Build history of the part. All positions in model axes, mm. Round coordinates to 2 decimals unless told otherwise and drop trailing zeros. Write each loop counter-clockwise with the first axis right and the second up, starting at its lowest first coordinate (ties: lowest second). Pieces come first, ordered by that corner, then holes. Notation, with made-up numbers: (29, -4) -> (53, -4) arc R23 cw to (53, 33) -> close; hole circle Ø3 at (23, 57). An arc over 180 degrees is marked (long way). Answer as CSV lines item,"result".
from build123d import *

# Parameters (mm, degrees)
BOSS_EXTRUDE1_START     = 92.868812
BOSS_EXTRUDE1_DEPTH     = 3.175
FILLET1_R               = 9.525
F_1_4_CLEARANCE_HOLE1_D = 6.7564


with BuildPart() as part:
    # Sketch2 → Boss-Extrude1 (new body)
    with BuildSketch(Plane(origin=(0, 0, 0), x_dir=(0, 0, -1), z_dir=(1, 0, 0)).offset(BOSS_EXTRUDE1_START)):
        with BuildLine():
            Line((-1159.986800073, 353.698023512), (-1134.923032257, 357.817191252))
            Line((-1134.923032257, 357.817191252), (-1092.891252047, 364.725009516))
            Line((-1092.891252047, 364.725009516), (-1111.090669966, 321.220387339))
            Line((-1111.090669966, 321.220387339), (-1120.893160292, 297.788119344))
            ThreePointArc((-1120.893160292, 297.788119344), (-1128.752566193, 291.984337623), (-1137.588017099, 296.1543437))
            Line((-1137.588017099, 296.1543437), (-1166.34986848, 338.989401064))
            ThreePointArc((-1166.34986848, 338.989401064), (-1167.184141053, 348.080982608), (-1159.986800073, 353.698023512))
        make_face()
    extrude(amount=BOSS_EXTRUDE1_DEPTH)

    # Fillet1
    fillet1_edges = [part.edges().sort_by_distance(p)[0] for p in [
        (94.456312, 364.725009516, 1092.891252047),
    ]]
    fillet(fillet1_edges, radius=FILLET1_R)

    # 1/4 Clearance Hole1 (through all)
    with Locations(Plane(origin=(96.043812484, 0, 0), x_dir=(0, 0, -1), z_dir=(1, 0, 0))):
        with Locations((-1133.378344355, 348.418278321), (-1158.442112171, 344.299110581), (-1129.68026079, 301.464053216), (-1119.877770464, 324.896321212)):
            Hole(F_1_4_CLEARANCE_HOLE1_D / 2)


solid = part.part
1. Probe line 1 along Z through (x, y) = (95.4, 346.5); line 2 along Z through (x, y) = (94.7, 348); line 3 along Y through (x, z) = (95.75, 1135.5). List the from-to ranges inside material, lowest first.
Results found:
line 1,"z = 1100.52 to 1130.6, 1136.16 to 1155.88, 1161 to 1167.71"
line 2,"z = 1099.89 to 1130.03, 1136.73 to 1167.22"
line 3,"y = 293.92 to 345.79, 351.05 to 357.72"
2. Cut at D-D, the plane z = 1131.5. Write the cut outline in (x, y).
Results found:
outline,"(92.87, 292.11) -> (96.04, 292.11) -> (96.04, 298.62) -> (92.87, 298.62) -> close; (92.87, 304.31) -> (96.04, 304.31) -> (96.04, 345.61) -> (92.87, 345.61) -> close; (92.87, 351.23) -> (96.04, 351.23) -> (96.04, 358.38) -> (92.87, 358.38) -> close"
3. Cut at B-B, the plane y = 350.5. Write the cut outline in (x, z), then the cut area to 3 significant figures.
Results found:
outline,"(92.87, 1099.01) -> (96.04, 1099.01) -> (96.04, 1130.72) -> (92.87, 1130.72) -> close; (92.87, 1136.04) -> (96.04, 1136.04) -> (96.04, 1165.67) -> (92.87, 1165.67) -> close"
area,"195 mm2"
4. Drop flat-ended pins along their axis: pin 1 Ø6 at (y, z) = (348.42, 1133.38) entering from +X; pin 2 Ø1 at (x, y) = (93, 317) entering from +Z. Give the stop position or say it passes through.
Results found:
pin 1,"passes through"
pin 2,"stops at z = 1151.92"
5. Cut at A-A, the plane z = 1156. Write the cut outline in (x, y), then the cut area to 3 significant figures.
Results found:
outline,"(92.87, 323.58) -> (96.04, 323.58) -> (96.04, 341.96) -> (92.87, 341.96) -> close; (92.87, 346.63) -> (96.04, 346.63) -> (96.04, 354.35) -> (92.87, 354.35) -> close"
area,"82.9 mm2"
6. Cut at C-C, the plane x = 93.9. Write the cut outline in (y, z) (3 decimals), then the cut area to 3 significant figures.
Results found:
outline,"(296.154, 1137.588) arc R9.525 ccw to (297.788, 1120.893) -> (348.862, 1099.527) arc R9.525 ccw to (361.936, 1109.859) -> (353.698, 1159.987) arc R9.525 ccw to (338.989, 1166.35) -> close; hole circle Ø6.756 at (301.464, 1129.68); hole circle Ø6.756 at (324.896, 1119.878); hole circle Ø6.756 at (344.299, 1158.442); hole circle Ø6.756 at (348.418, 1133.378)"
area,"2,840 mm2"
